Geometry check sheet. Reference: the model listing, model coordinates, mm. Coordinates: 2 decimals unless noted, no trailing zeros. Loops run counter-clockwise (first coordinate to the right, second up) from the corner with the lowest first, then second, coordinate; pieces in that order, holes last. Notation, with made-up numbers: (47.25, 36) -> (83.25, 36) arc R35 cw to (83.25, 74) -> close; hole circle Ø10 at (-8, -33). An arc over 180 degrees is marked (long way). Answer as a JSON object with one key per item and string values.
Autodesk Inventor part; units mm, degrees
ref_plane "YZ Plane" through (0, 0, 0) normal (1, 0, 0) x (0, 1, 0)
ref_plane "XY Plane" through (0, 0, 0) normal (0, 0, 1) x (1, 0, 0)
sketch "Sketch2" plane through (0, 0, 0) normal (0, 0, 1) x (1, 0, 0)
  line L0 (-75, -25) -> (75, -25)
  line L1 (75, -25) -> (75, 25)
  line L2 (75, 25) -> (-75, 25)
  line L3 (-75, 25) -> (-75, -25)
  line L4 (-75, -25) -> (75, 25) construction
  line L5 (75, -25) -> (-75, 25) construction
  point P0 (0, 0)
  dimension "d1" = 150
  dimension "d2" = 50
extrude "Extrusion1" add sketch "Sketch2" along normal mid plane 10
sketch "Sketch3" plane through (0, 0, 5) normal (0, 0, 1) x (1, 0, 0)
  line L0 (-75, 25) -> (-75, -25)
  line L1 (75, 25) -> (-75, 25)
  point P0 (0, 0)
  point P1 (-65, 0)
  dimension "d40" = 10
  dimension "d43" = 25
hole "Hole1" at (-65, 0, 5) direction (0, 0, -1) diameter 4.134 depth 14.2 tip angle 118
sketch "Sketch4" plane through (0, 0, 5) normal (0, 0, 1) x (1, 0, 0)
  line L0 (-75, 25) -> (-75, -25)
  line L1 (75, 25) -> (-75, 25)
  point P0 (0, 0)
  point P1 (-45, 5)
  dimension "d41" = 30
  dimension "d42" = 20
hole "Hole2" at (-45, 5, 5) direction (0, 0, -1) diameter 4.917 depth 17.1 tip angle 118
sketch "Sketch5" plane through (0, 0, 5) normal (0, 0, 1) x (1, 0, 0)
  line L0 (-75, 25) -> (-75, -25)
  line L1 (75, 25) -> (-75, 25)
  point P0 (0, 0)
  point P1 (-24, 5)
  dimension "d44" = 51
  dimension "d45" = 20
hole "Hole3" at (-24, 5, 5) direction (0, 0, -1) diameter 6.647 depth 22.2 tip angle 118
sketch "Sketch6" plane through (0, 0, 5) normal (0, 0, 1) x (1, 0, 0)
  line L0 (-75, 25) -> (-75, -25)
  line L1 (75, 25) -> (-75, 25)
  point P0 (0, 0)
  point P1 (5, 5)
  dimension "d46" = 80
  dimension "d47" = 20
hole "Hole4" at (5, 5, 5) direction (0, 0, -1) diameter 6 depth 14.2 tip angle 118
sketch "Sketch7" plane through (0, 0, 5) normal (0, 0, 1) x (1, 0, 0)
  line L0 (-75, 25) -> (-75, -25)
  line L1 (75, 25) -> (-75, 25)
  point P0 (0, 0)
  point P1 (25, 5)
  dimension "d48" = 100
  dimension "d49" = 20
hole "Hole5" at (25, 5, 5) direction (0, 0, -1) diameter 10 depth 14.2 tip angle 118
pattern_linear "Rectangular Pattern1" count 3 spacing 11 along (0, -1, 0) of "Hole1" first direction both ways yes
mirror "Mirror1" about plane through (0, 0, 0) normal (0, 1, 0) of "Hole2"
pattern_linear "Rectangular Pattern2" count 3 spacing 10 along (0, -1, 0) of "Hole4"
ref_plane "Work Plane1" through (0, -2.25, 0) normal (0, 1, 0) x (-1, 0, 0)
mirror "Mirror3" about plane through (0, -2.25, 0) normal (0, 1, 0) of "Hole3"
pattern_linear "Rectangular Pattern3" count 2 spacing 20 along (0, -1, 0) of "Hole5"
ref_plane "Work Plane2" through (0, -2.25, 0) normal (0, 1, 0) x (-1, 0, 0)
properties part number "홀간 거리 확인 파트-4" material "SS400"
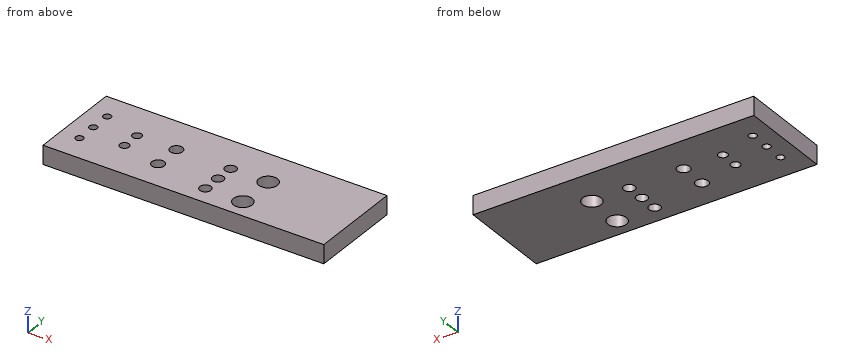
1. Thickness scan on probe 1 along Y at (x, z) = (-24, -0.25); probe 2 along X at (y, z) = (-5, -2.5); probe 3 along X at (y, z) = (6, -0.75). Record the ranges inside material, lowest first. Write a range as from..to.
Evaluation:
{"probe 1": "y = -25..-12.82, -6.18..1.68, 8.32..25", "probe 2": "x = -75..-47.46, -42.54..2, 8..75", "probe 3": "x = -75..-47.25, -42.75..-27.17, -20.83..2.17, 7.83..20.1, 29.9..75"}
2. Section check B-B, the plane x = 25. Record the boundary of the cut face in (y, z).
Evaluation:
{"outline": "(-25, -5) -> (-20, -5) -> (-20, 5) -> (-25, 5) -> close; (-10, -5) -> (0, -5) -> (0, 5) -> (-10, 5) -> close; (10, -5) -> (25, -5) -> (25, 5) -> (10, 5) -> close"}
3. Section check C-C, the plane z = 0.25. State how many separate pieces and enclosed holes the cut face has, then the cut area to 3 significant figures.
Evaluation:
{"separate pieces": "1", "enclosed holes": "12", "area": "7,110 mm^2"}
4. Section check A-A, the plane y = -15. Record the boundary of the cut face in (x, z).
Evaluation:
{"outline": "(-75, -5) -> (2, -5) -> (2, 5) -> (-75, 5) -> close; (8, -5) -> (20, -5) -> (20, 5) -> (8, 5) -> close; (30, -5) -> (75, -5) -> (75, 5) -> (30, 5) -> close"}
5. Depth check by flat-ended pin: P1, Ø8, axis at x = 25, y = 5, coming from the -Z side; P2, Ø8, axis at x = 5, y = -15, coming from the -Z side. Enter the tip coordinate at first touch or a pass-through.
Evaluation:
{"P1": "passes through", "P2": "stops at z = -5"}
6. Section check D-D, the plane x = -65. Record the boundary of the cut face in (y, z), then the cut area to 3 significant figures.
Evaluation:
{"outline": "(-25, -5) -> (-13.07, -5) -> (-13.07, 5) -> (-25, 5) -> close; (-8.93, -5) -> (-2.07, -5) -> (-2.07, 5) -> (-8.93, 5) -> close; (2.07, -5) -> (8.93, -5) -> (8.93, 5) -> (2.07, 5) -> close; (13.07, -5) -> (25, -5) -> (25, 5) -> (13.07, 5) -> close", "area": "376 mm^2"}
